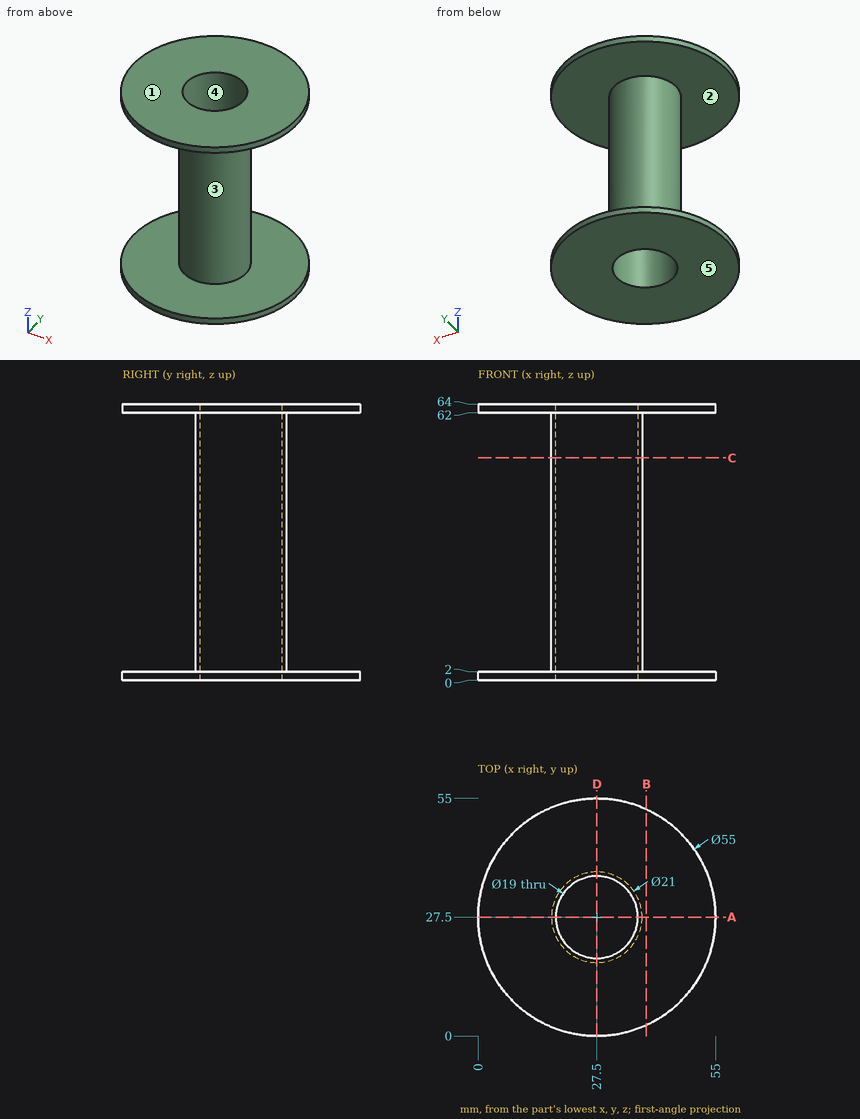
Verification items for this drawing (mm, ordinates from the low corner). A direction names the side the tool comes from. Coordinates: 2 decimals unless noted, no trailing zeros. Write each loop counter-clockwise with the first axis right and the second up, starting at its lowest first coordinate (ties: lowest second). Pieces come first, ordered by that corner, then holes. Notation, with made-up numbers: (19, 61.5) -> (43, 61.5) arc R24 cw to (43, 71.5) -> close; hole circle Ø4 at (81, 71). An arc over 180 degrees is marked (long way). Use CSV: the item, a comma, the result in double quotes. Start each with the question number.
Item 1: Set-up check for the marked faces 1 and 2: record each of +Z, -Z, +X, -X, +Y, -Y from which the full face is reachable in a straight line by a thin tool's end or side.
Item 2: Mould release check, pull along Z, two halves, no side actions. Record for the marked faces 3, 4 and 5: released by +Z, released by -Z, zero draft, split by the parting line, or undercut.
Item 3: Cross-section at B-B, the plane x = 39. Record the cut outline in (y, z), plus the area to 3 significant figures.
Item 4: Depth check by flat-ended pin: pin 1 Ø4 at (y, z) = (36, 48) entering from +X; pin 2 Ø3 at (y, z) = (14, 7.5) entering from +X; pin 3 Ø2 at (y, z) = (22.5, 21) entering from -X; pin 4 Ø6 at (y, z) = (28.5, 56.5) entering from +X. Enter the tip coordinate at first touch or a pass-through.
Item 5: Cross-section at C-C, the plane z = 51.5. Record the cut outline in (x, y).
Item 6: Cross-section at A-A, the plane y = 27.5. Record the cut outline in (x, z).
Item 7: Thickness scan on line 1 (Y direction, x = 27.5, z = 17.5); line 2 (Z direction, x = 31, y = 44); line 3 (X direction, y = 27, z = 22). Record the ranges inside material, lowest first.
Answers:
1,face 1,"+Z, +X, -X, +Y, -Y"
1,face 2,"none"
2,face 3,"undercut"
2,face 4,"zero draft"
2,face 5,"released by -Z"
3,outline,"(2.52, 0) -> (52.48, 0) -> (52.48, 2) -> (2.52, 2) -> close; (2.52, 62) -> (52.48, 62) -> (52.48, 64) -> (2.52, 64) -> close"
3,area,"200 mm^2"
4,pin 1,"x = 35.75"
4,pin 2,"through"
4,pin 3,"x = 17.79"
4,pin 4,"x = 38"
5,outline,"circle Ø21 at (27.5, 27.5); hole circle Ø19 at (27.5, 27.5)"
6,outline,"(0, 0) -> (18, 0) -> (18, 64) -> (0, 64) -> (0, 62) -> (17, 62) -> (17, 2) -> (0, 2) -> close; (37, 0) -> (55, 0) -> (55, 2) -> (38, 2) -> (38, 62) -> (55, 62) -> (55, 64) -> (37, 64) -> close"
7,line 1,"17 to 18, 37 to 38"
7,line 2,"0 to 2, 62 to 64"
7,line 3,"17.01 to 18.01, 36.99 to 37.99"
